from build123d import *

# Parameters (mm, degrees)
BOSS_EXTRUDE1_DEPTH = 1.8
SKETCH2_W           = 6
SKETCH2_H           = 10
BOSS_EXTRUDE2_DEPTH = 0.75
SKETCH3_W           = 2.7
SKETCH3_H           = 3.3
BOSS_EXTRUDE3_DEPTH = 0.9
SKETCH4_R           = 0.85
BOSS_EXTRUDE4_DEPTH = 1.6
SKETCH5_W           = 2.2
SKETCH5_H           = 1.35
BOSS_EXTRUDE5_DEPTH = 2
SKETCH7_W           = 1.65
SKETCH7_H           = 3.3
CUT_EXTRUDE2_DEPTH  = 0.4
CHAMFER1_SIZE       = 0.2
SKETCH9_R           = 0.4
CUT_EXTRUDE4_DEPTH  = 0.2


with BuildPart() as part:
    # Sketch1 → Boss-Extrude1 (new body)
    with BuildSketch(Plane(origin=(0, 0, 0), x_dir=(1, 0, 0), z_dir=(0, 1, 0))):
        Polygon((-1.4, 3), (-1.4, 0), (-1.975, 0), (-1.975, -1.5), (1.975, -1.5), (1.975, 0), (1.4, 0), (1.4, 3), (3, 3), (3, -7), (-3, -7), (-3, 3), align=None)
    extrude(amount=BOSS_EXTRUDE1_DEPTH)

    # Sketch2 → Boss-Extrude2 (add)
    with BuildSketch(Plane.XZ):
        with Locations((0, 2)):
            Rectangle(SKETCH2_W, SKETCH2_H)
    extrude(amount=BOSS_EXTRUDE2_DEPTH)

    # Sketch3 → Boss-Extrude3 (add)
    with BuildSketch(Plane(origin=(0, 1.8, 0), x_dir=(1, 0, 0), z_dir=(0, 1, 0))):
        with Locations((0, -4)):
            Rectangle(SKETCH3_W, SKETCH3_H)
    extrude(amount=BOSS_EXTRUDE3_DEPTH)

    # Sketch4 → Boss-Extrude4 (add)
    with BuildSketch(Plane(origin=(0, 2.7, 0), x_dir=(1, 0, 0), z_dir=(0, 1, 0))):
        with Locations(Location((0, -4, 0), (0, 0, 270))):
            Circle(SKETCH4_R)
    extrude(amount=BOSS_EXTRUDE4_DEPTH)

    # Sketch5 → Boss-Extrude5 (add)
    with BuildSketch(Plane(origin=(0, 1.8, 0), x_dir=(1, 0, 0), z_dir=(0, 1, 0))):
        with Locations((0, -6.325)):
            Rectangle(SKETCH5_W, SKETCH5_H)
    extrude(amount=BOSS_EXTRUDE5_DEPTH)

    # Sketch7 → Cut-Extrude2 (cut)
    with BuildSketch(Plane(origin=(0, 1.8, 0), x_dir=(1, 0, 0), z_dir=(0, 1, 0))):
        with Locations((-2.175, -4)):
            Rectangle(SKETCH7_W, SKETCH7_H)
        with Locations((2.175, -4)):
            Rectangle(SKETCH7_W, SKETCH7_H)
    extrude(amount=-CUT_EXTRUDE2_DEPTH, mode=Mode.SUBTRACT)

    # Chamfer1
    chamfer1_edges = [part.edges().sort_by_distance(p)[0] for p in [
        (-2.175, 1.8, 2.35),
        (-2.175, 1.8, 5.65),
        (2.175, 1.8, 5.65),
        (2.175, 1.8, 2.35),
    ]]
    chamfer(chamfer1_edges, length=CHAMFER1_SIZE)

    # Sketch9 → Cut-Extrude4 (cut)
    with BuildSketch(Plane(origin=(3, 0, 0), x_dir=(0, 0, -1), z_dir=(1, 0, 0))):
        with Locations((1.9, 0.8)):
            Circle(SKETCH9_R)
    cut_extrude4 = extrude(amount=-CUT_EXTRUDE4_DEPTH, mode=Mode.SUBTRACT)

    # Mirror1: Cut-Extrude4 across plane
    add(cut_extrude4.mirror(Plane(origin=(0, 0, 0), x_dir=(0, 0, 1), z_dir=(1, 0, 0))), mode=Mode.SUBTRACT)


solid = part.part
Here's how the part is built. I have some questions about the finished solid (model axes, mm). A direction names the side the tool comes from. Round coordinates to 2 decimals unless told otherwise and drop trailing zeros. Order: outer loops, then holes, each group sorted by start corner. A loop starts at its lowest first (then second) coordinate and runs counter-clockwise, first axis right, second up. Notation, with made-up numbers: M 41.25,52 L 95.25,52 A24 ccw 95.25,80 Z; hole C -2.75,-17 d2. An arc over 180 degrees is marked long. Return JSON: item names as keys, results as strings. Group by question number.
1. On a 3-axis mill with a long thin cutter (end or side, diameter ignored), from which of +Z, -Z, +X, -X, +Y, -Y can I reach the whole of each face in a straight line? I mean faces 1 (the face through (1.1, 3, 6)), 2 (the face through (-1.4, 1, -2)), 3 (the face through (1.975, 1, 1)). Say none if no direction works.
2. If we section it at A-A on y = 3.3: List the corners of the cut face in (x, z) for me.
3. If we section it at C-C on x = 0: List the corners of the cut face in (y, z) for me.
4. If we section it at D-D on z = -1.9: List the corners of the cut face in (x, y) for me, then the cut area to 3 significant figures.
5. If we section it at B-B on z = 4: List the corners of the cut face in (x, y) for me.
6. Please list where these lines run through material, in increasing order: probe 1 along Z at (x, y) = (1.55, 1.2); probe 2 along Y at (x, z) = (2.9, -1.9); probe 3 along X at (y, z) = (1, 0.5) (3 decimals).
7. If we mould it in two halves opening along X, with no side actions, what happens to faces 4 (the face through (-1.975, 1, 1)), 5 (the face through (-2, 1.4, 4)), 6 (the face through (1.35, 2, 4)), 7 (the face through (-3, 1, 2))? For each: pulls with the +X half, pulls with the -X half, needs draft (parallel to the pull), parting line crosses it, or undercut.
8. I'm going to push flat-ended pins straight in: pin 1 Ø1.1 at (x, z) = (-0.5, 6) entering from +Y; pin 2 Ø0.7 at (x, z) = (-1.5, 6) entering from +Y; pin 3 Ø1 at (y, z) = (2, 3.5) entering from +X. Where does each tip first touch, or does it pass through?
Reply:
{
 "1": {"face 1": "+Z, +X, +Y", "face 2": "-Z, +Y", "face 3": "+Y"},
 "2": {"outline": "M -1.1,5.65 L 1.1,5.65 L 1.1,7 L -1.1,7 Z; C 0,4 d1.7"},
 "3": {"outline": "M -0.75,-3 L 0,-3 L 0,1.5 L 1.8,1.5 L 1.8,2.35 L 2.7,2.35 L 2.7,3.15 L 4.3,3.15 L 4.3,4.85 L 2.7,4.85 L 2.7,5.65 L 3.8,5.65 L 3.8,7 L -0.75,7 Z"},
 "4": {"outline": "M -3,-0.75 L 3,-0.75 L 3,0.4 L 2.8,0.4 L 2.8,1.2 L 3,1.2 L 3,1.8 L 1.4,1.8 L 1.4,0 L -1.4,0 L -1.4,1.8 L -3,1.8 L -3,1.2 L -2.8,1.2 L -2.8,0.4 L -3,0.4 Z", "area": "9.94 mm^2"},
 "5": {"outline": "M -3,-0.75 L 3,-0.75 L 3,1.4 L 1.35,1.4 L 1.35,2.7 L 0.85,2.7 L 0.85,4.3 L -0.85,4.3 L -0.85,2.7 L -1.35,2.7 L -1.35,1.4 L -3,1.4 Z"},
 "6": {"probe 1": "-3 to 0, 1.5 to 7", "probe 2": "-0.75 to 0.4, 1.2 to 1.8", "probe 3": "-3 to -1.975, 1.975 to 3"},
 "7": {"face 4": "undercut", "face 5": "needs draft", "face 6": "pulls with the +X half", "face 7": "pulls with the -X half"},
 "8": {"pin 1": "y = 3.8", "pin 2": "y = 1.8", "pin 3": "x = 1.35"}
}
